from build123d import *

# Parameters (mm, degrees)
F0_W     = 20
F0_H     = 20
F0_R     = 1.75
F1_DEPTH = 3.5
F2_R     = 3
F3_DEPTH = 2
F4_W     = 3
F4_H     = 2
F4_H_2   = 4
F5_DEPTH = 15
F6_W     = 5.121377
F6_H     = 27.98892
F7_DEPTH = 25


with BuildPart() as f1:
    # F0 (on Front) → F1 (new body)
    with BuildSketch(Plane.XZ):
        with Locations((10, 10)):
            Rectangle(F0_W, F0_H)
        with Locations((10, 10)):
            Circle(F0_R, mode=Mode.SUBTRACT)
    extrude(amount=F1_DEPTH)

    # F2 (on face) → F3 (cut)
    with BuildSketch(Plane.XZ.offset(3.5)):
        with Locations((10, 10)):
            Circle(F2_R)
    extrude(amount=-F3_DEPTH, mode=Mode.SUBTRACT)

    # F4 (on face) → F5 (join)
    with BuildSketch(Plane(origin=(0, 0, 0), x_dir=(-1, 0, 0), z_dir=(0, 1, 0))):
        with Locations((-1.5, -1)):
            Rectangle(F4_W, F4_H)
        with Locations((-10, 20)):
            Rectangle(F4_W, F4_H_2)
        with Locations((-1.5, 0)):
            Rectangle(F4_W, F4_H_2)
        with Locations((-18.5, 0)):
            Rectangle(F4_W, F4_H_2)
    extrude(amount=-F5_DEPTH)

    # F6 (on face) → F7 (cut)
    with BuildSketch(Plane(origin=(0, 0, 0), x_dir=(0, -1, 0), z_dir=(-1, 0, 0))):
        Polygon((7.894673, 21), (6.5, 20.877982), (8.417426, -1.038301), (9.812099, -0.916283), align=None)
        with Locations((14.084454, 9.811153)):
            Rectangle(F6_W, F6_H)
    extrude(amount=-F7_DEPTH, mode=Mode.SUBTRACT)


solid = f1.part
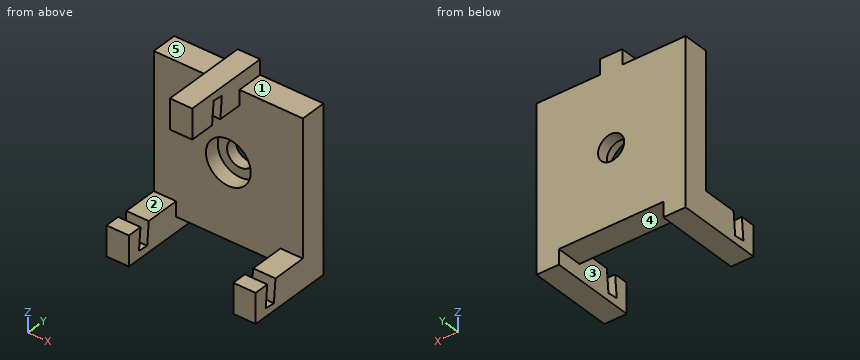
Can you work these out from the model? Positions are in its coordinate system, mm. Face numbers are marked on the shaded views. A direction names the side the tool comes from. Give positions to 0.01 mm unless a question says otherwise; leave off trailing zeros. Write each loop counter-clockwise with the first axis right and the second up, starting at its lowest first coordinate (ties: lowest second). Pieces come first, ordered by that corner, then holes. Notation, with made-up numbers: M 73.25,23 L 126.25,23 A31 ccw 126.25,54 Z; hole C 46.5,61 d4. An arc over 180 degrees is marked long. Answer in a Markdown table with one row per item. Add a question column.
Item 1: Imagine slicing it at C-C, the plane x = 18.5. Write out the boundary of the cut face in (y, z), plus the area to 3 significant figures.
Item 2: On a 3-axis mill with a long thin cutter (end or side, diameter ignored), from which of +Z, -Z, +X, -X, +Y, -Y can I reach the whole of each face in a straight line? I mean the marked faces 1, 2, 3, 4 and 5. Say none if no direction works.
Item 3: Imagine slicing it at B-B, the plane x = 10. Write out the boundary of the cut face in (y, z), plus the area to 3 significant figures.
Item 4: For pin 1 Ø1.6 at (x, y) = (2, -10.5) entering from +Z; pin 2 Ø6 at (x, z) = (17, 9.5) entering from +Y; pin 3 Ø4.5 at (y, z) = (-6, 19) entering from -X; pin 4 Ø1.5 at (x, y) = (9.5, -5.5) entering from -Z, each with a flat end and sliding along its axis, tell me the tip position at first contact or that it passes through.
Item 5: Imagine slicing it at A-A, the plane z = 10. Write out the boundary of the cut face in (x, y), plus the area to 4 significant figures.
Item 6: Imagine slicing it at D-D, the plane z = 2.5. Write out the boundary of the cut face in (x, y).
Item 7: Please list where these lines run through material, in increasing order: L1, parallel to Z at x = 10, y = -0.9; L2, parallel to Z at x = 10, y = -2.7; L3, parallel to X at y = -0.4, z = 10.
Evaluation:
| question | item | result |
|---|---|---|
| 1 | outline | M -11.52,-2 L 0,-2 L 0,20 L -3.5,20 L -3.5,2 L -8.15,2 L -8.42,-1.04 L -9.81,-0.92 L -9.56,2 L -11.52,2 Z |
| 1 | area | 105 mm² |
| 2 | face 1 | +Z, +X, +Y, -Y |
| 2 | face 2 | +Z, +X, -X, -Y |
| 2 | face 3 | -Z, -Y |
| 2 | face 4 | -Z, +Y, -Y |
| 2 | face 5 | +Z, -X, +Y, -Y |
| 3 | outline | M -11.52,18 L -8.16,18 L -7.89,21 L -6.5,20.88 L -6.75,18 L -3.5,18 L -3.5,13 L -1.5,13 L -1.5,11.75 L 0,11.75 L 0,22 L -11.52,22 Z; M -3.5,0 L 0,0 L 0,8.25 L -1.5,8.25 L -1.5,7 L -3.5,7 Z |
| 3 | area | 87.7 mm² |
| 4 | pin 1 | stops at z = 2 |
| 4 | pin 2 | stops at y = 0 |
| 4 | pin 3 | stops at x = 8.5 |
| 4 | pin 4 | stops at z = 18 |
| 5 | outline | M 0,-3.5 L 7,-3.5 L 7,-1.5 L 8.25,-1.5 L 8.25,0 L 0,0 Z; M 11.75,-1.5 L 13,-1.5 L 13,-3.5 L 20,-3.5 L 20,0 L 11.75,0 Z |
| 5 | area | 52.75 mm² |
| 6 | outline | M 0,-3.5 L 20,-3.5 L 20,0 L 0,0 Z |
| 7 | L1 | z = 0 to 8.25, 11.75 to 22 |
| 7 | L2 | z = 0 to 7, 13 to 22 |
| 7 | L3 | x = 0 to 8.25, 11.75 to 20 |
